```python
from build123d import *

# Parameters (mm, degrees)
F1_DEPTH = 6.35


with BuildPart() as f1:
    # F0 (on Top) → F1 (new body)
    with BuildSketch(Plane.XY):
        with BuildLine():
            ThreePointArc((0, 12.7), (-4.801349, 11.757425), (-8.89, 9.069614))
            ThreePointArc((-8.89, 9.069614), (0, -12.7), (8.89, 9.069614))
            ThreePointArc((8.89, 9.069614), (4.801349, 11.757425), (0, 12.7))
        make_face()
        with BuildLine():
            Line((-8.89, 61.97625), (-8.89, 9.069614))
            ThreePointArc((-8.89, 9.069614), (-4.801349, 11.757425), (0, 12.7))
            ThreePointArc((0, 12.7), (4.801349, 11.757425), (8.89, 9.069614))
            Line((8.89, 9.069614), (8.89, 44.19625))
            ThreePointArc((8.89, 44.19625), (10.749872, 48.686378), (15.24, 50.54625))
            Line((15.24, 50.54625), (34.68042, 50.54625))
            ThreePointArc((34.68042, 50.54625), (47.625, 59.43625), (34.68042, 68.32625))
            Line((34.68042, 68.32625), (-2.54, 68.32625))
            ThreePointArc((-2.54, 68.32625), (-7.030128, 66.466378), (-8.89, 61.97625))
        make_face()
    extrude(amount=F1_DEPTH)


solid = f1.part
```
Source: CAD feature listing. Evaluate the final solid. Frame: model axes, mm. A direction names the side the tool comes from. Round coordinates to 2 decimals unless told otherwise and drop trailing zeros. Loops run counter-clockwise (first coordinate to the right, second up) from the corner with the lowest first, then second, coordinate; pieces in that order, holes last. Notation, with made-up numbers: (65, -39) - (92, -39) arc R12 cw to (92, -16) - close; hole circle Ø4 at (14.5, -36.5). An arc over 180 degrees is marked (long way). Use CSV: the item, a comma, the result in double quotes.
Q1. Mould query, pull axis Y, two halves, no side actions, for faces 4 (the flat face through (16, 68.326, 3)), 5 (the cylindrical face through (10.701, 48.637, 3.131)), 6 (the flat face through (-8.89, 36, 3)). Classes: pulls with the +Y half, pulls with the -Y half, needs draft (parallel to the pull), parting line crosses it, or undercut.
Reported:
face 4,"pulls with the +Y half"
face 5,"undercut"
face 6,"needs draft"
Q2. Section query A-A, the plane z = 5.25. Output: boundary loops of the cut face in (x, y) (3 decimals).
Reported:
outline,"(-8.89, 9.07) arc R12.7 ccw (long way) to (8.89, 9.07) - (8.89, 44.196) arc R6.35 cw to (15.24, 50.546) - (34.68, 50.546) arc R9.525 ccw (long way) to (34.68, 68.326) - (-2.54, 68.326) arc R6.35 ccw to (-8.89, 61.976) - close"
Q3. Section query B-B, the plane y = 0. Output: boundary loops of the cut face in (x, z), then the cut area to 3 significant figures.
Reported:
outline,"(-12.7, 0) - (12.7, 0) - (12.7, 6.35) - (-12.7, 6.35) - close"
area,"161 mm^2"
Q4. Reachability of faces 1 (the flat face through (4, 38, 0)), 2 (the flat face through (8.89, 26, 3)), 3 (the flat face through (25, 50.546, 3)) from +Z, -Z, +X, -X, +Y, -Y: full face, straight path, thin tool, end or side. Return the list, or none.
Reported:
face 1,"-Z, +X, -X, +Y, -Y"
face 2,"+Z, -Z, +X"
face 3,"+Z, -Z, -Y"
Q5. Ray query, line 1 along X through (y, z) = (38.5, 4); line 2 along Y through (x, z) = (22.5, 6); line 3 along Y through (x, z) = (10.5, 3). Return the intervals inside material, ascending.
Reported:
line 1,"-8.89 to 8.89"
line 2,"50.55 to 68.33"
line 3,"-7.14 to 7.14, 48.42 to 68.33"
Q6. Pin query (flat end, axial travel): pin 1 Ø3 at (x, z) = (17, 4.5) entering from +Y; pin 2 Ø1.5 at (x, z) = (32.5, 2) entering from -Y; pin 3 Ø1.5 at (y, z) = (55, 5.5) entering from +X. Return the tip coordinate at first contact, or that it passes through.
Reported:
pin 1,"y = 68.33"
pin 2,"y = 50.55"
pin 3,"x = 46.88"
Q7. Section query C-C, the plane x = 33. Output: boundary loops of the cut face in (y, z).
Reported:
outline,"(50.55, 0) - (68.33, 0) - (68.33, 6.35) - (50.55, 6.35) - close"
